Check sheet for the drawn part. Datum: minimum x, y, z corner. Units: mm. Coordinates: 2 decimals unless noted, no trailing zeros. Order: outer loops, then holes, each group sorted by start corner. A loop starts at its lowest first (then second) coordinate and runs counter-clockwise, first axis right, second up. Notation, with made-up numbers: (-6, 79.25) - (6, 79.25) arc R35 cw to (6, 113.25) - close; hole circle Ø6 at (6, -32.75). An arc over 180 degrees is marked (long way). Answer as CSV lines item,"result". Start each with the question number.
1. Material ranges on L1, parallel to Y at x = 1.45, z = 30; L2, parallel to Y at x = 0.1, z = 7; L3, parallel to Z at x = 0.2, y = 4, recorded low to high. Write a range as [from, to].
2. Section check B-B (x = 1.35). Record the cut outline in (y, z), and give its area (4 significant figures).
3. Section check A-A (z = 18). Record the cut outline in (x, y).
4. Section check C-C (y = 13.5). Record the cut outline in (x, z).
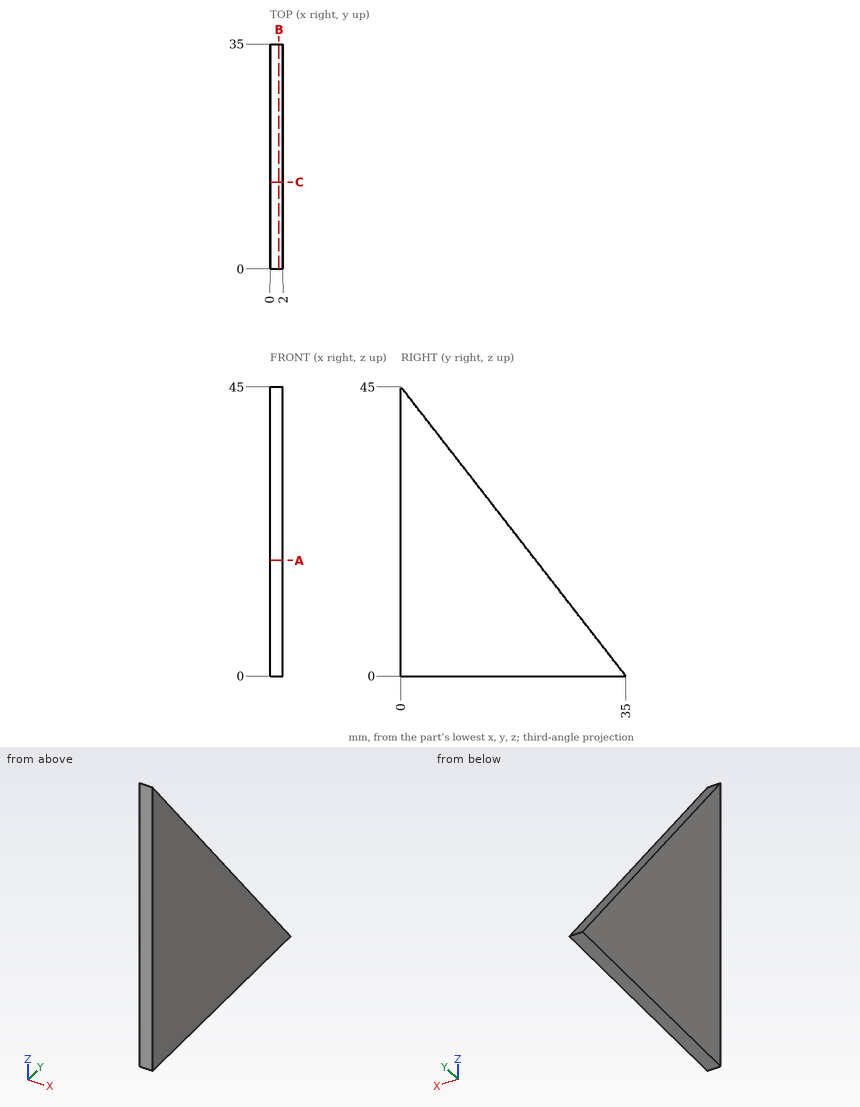
Evaluation:
1,L1,"y = [0, 11.67]"
1,L2,"y = [0, 29.56]"
1,L3,"z = [0, 39.86]"
2,outline,"(0, 0) - (35, 0) - (0, 45) - close"
2,area,"787.5 mm²"
3,outline,"(0, 0) - (2, 0) - (2, 21) - (0, 21) - close"
4,outline,"(0, 0) - (2, 0) - (2, 27.64) - (0, 27.64) - close"
